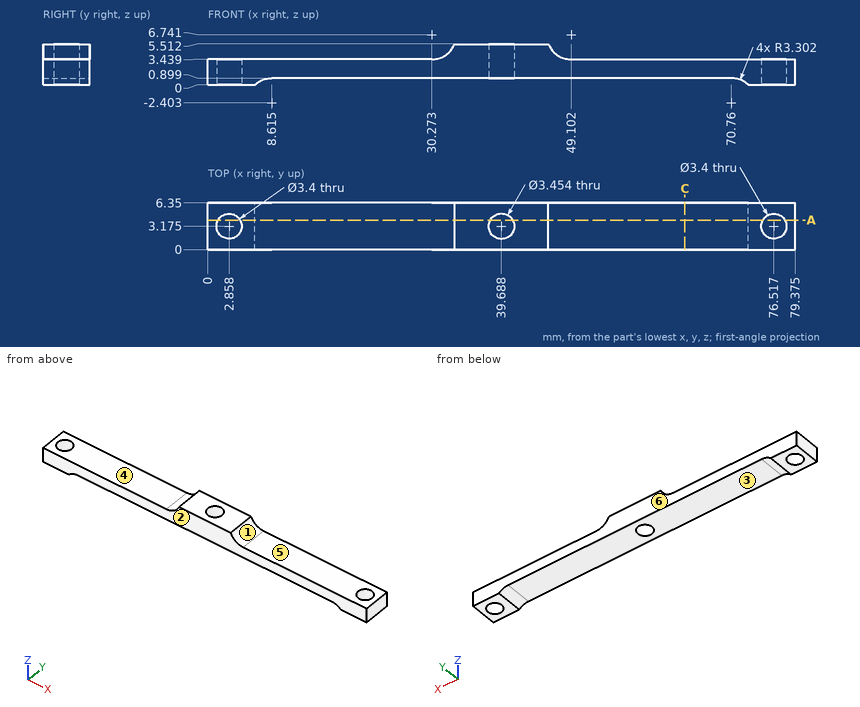
Input: dimensioned drawing with shaded views. Units: mm. Origin: part minimum x, y, z. A direction names the side the tool comes from. Coordinates: 2 decimals unless noted, no trailing zeros. Loops run counter-clockwise (first coordinate to the right, second up) from the corner with the lowest first, then second, coordinate; pieces in that order, holes last. Notation, with made-up numbers: (78, 60) -> (127, 60) arc R25 ccw to (127, 74) -> close; hole circle Ø4 at (9, 78.25). An arc over 180 degrees is marked (long way). Use a Markdown table: item, result. Add a question column.
(1) Line query: line 1 along X through (y, z) = (3, 1.7) (1 decimal); line 2 along X through (y, z) = (3.75, 1.05) (1 decimal); line 3 along Z through (x, y) = (53.5, 6). Output: solid intervals per line, ascending.
(2) Pin query (flat end, axial travel): pin 1 Ø3 at (y, z) = (2, 2.5) entering from -X; pin 2 Ø1.5 at (x, y) = (29, 2.5) entering from -Z; pin 3 Ø2.5 at (x, y) = (76.52, 3.18) entering from +Z; pin 4 Ø3 at (x, y) = (9, 3) entering from +Z. Return the tip coordinate at first contact, or that it passes through.
(3) Section query A-A, the plane y = 4. State how many separate pieces and enclosed holes the cut face has, plus the area to 3 significant figures.
(4) Access query for the marked faces 4, 5 and 6. Directions: +Z, -Z, +X, -X, +Y, -Y. A direction counts if a zero-diameter tool reaches every point of the face in a straight line with its end or side. Return the directions, or none.
(5) Section query C-C, the plane x = 64.5. Return loops of the section in (y, z), plus the area to 3 significant figures.
(6) Mould query, pull axis X, two halves, no side actions, for the marked faces 1, 2 and 3. Classes: pulls with the +X half, pulls with the -X half, needs draft (parallel to the pull), parting line crosses it, or undercut.
Answer:
| question | item | result |
|---|---|---|
| 1 | line 1 | x = 0 to 1.2, 4.5 to 38, 41.4 to 74.8, 78.2 to 79.4 |
| 1 | line 2 | x = 0 to 1.3, 4.5 to 38.1, 41.3 to 74.9, 78.1 to 79.4 |
| 1 | line 3 | z = 0.9 to 3.44 |
| 2 | pin 1 | stops at x = 0 |
| 2 | pin 2 | stops at z = 0.9 |
| 2 | pin 3 | passes through |
| 2 | pin 4 | stops at z = 3.44 |
| 3 | separate pieces | 4 |
| 3 | enclosed holes | 0 |
| 3 | area | 210 mm^2 |
| 4 | face 4 | +Z, -X, +Y, -Y |
| 4 | face 5 | +Z, +X, +Y, -Y |
| 4 | face 6 | +Z, -Z, +X, -X, +Y |
| 5 | outline | (0, 0.9) -> (6.35, 0.9) -> (6.35, 3.44) -> (0, 3.44) -> close |
| 5 | area | 16.1 mm^2 |
| 6 | face 1 | pulls with the +X half |
| 6 | face 2 | needs draft |
| 6 | face 3 | undercut |
